Autodesk Inventor part; units mm, degrees
ref_plane "YZ Plane" through (0, 0, 0) normal (1, 0, 0) x (0, 1, 0)
ref_plane "XZ Plane" through (0, 0, 0) normal (0, 1, 0) x (-1, 0, 0)
ref_plane "XY Plane" through (0, 0, 0) normal (0, 0, 1) x (1, 0, 0)
sketch "Sketch1" plane through (0, 0, 0) normal (0, 1, 0) x (-1, 0, 0)
  line L0 (-29, 41.5) -> (29, 41.5)
  line L1 (29, 41.5) -> (29, -41.5)
  line L2 (29, -41.5) -> (-29, -41.5)
  line L3 (-29, -41.5) -> (-29, 41.5)
  line L4 (-29, 41.5) -> (29, -41.5) construction
  line L5 (29, 41.5) -> (-29, -41.5) construction
  point P0 (0, 0)
  dimension "d0" = 83
  dimension "d1" = 58
extrude "Extrusion1" add sketch "Sketch1" along normal blind 1.5
sketch "Sketch2" plane through (0, 1.5, 0) normal (0, 1, 0) x (1, 0, 0)
  line L0 (-29, 41.5) -> (-29, -41.5)
  point P0 (0, 0)
  point P1 (-24.75, 5.75)
  point P2 (-24.75, -4.25)
  point P3 (-29, 0)
  dimension "d11" = 10
  dimension "d12" = 4.25
  dimension "d13" = 4.25
  dimension "d14" = 5.75
hole "Hole1" at (-24.75, 1.5, -5.75) at (-24.75, 1.5, 4.25) direction (0, -1, 0) diameter 2 end through all
properties part number "pcb" material "PBT Plastic"
Read the model definition and answer for the solid it produces. Units are mm, in the model's axes. Coordinates: 2 decimals unless noted, no trailing zeros. Write each loop counter-clockwise with the first axis right and the second up, starting at its lowest first coordinate (ties: lowest second). Pieces come first, ordered by that corner, then holes. Notation, with made-up numbers: (-22.75, 23.25) - (12.25, 23.25) arc R27 ccw to (12.25, 58.25) - close; hole circle Ø4 at (35.5, 43.25). An arc over 180 degrees is marked (long way). Answer as a JSON object with one key per item and string values. Group by question number.
1. Consider L1, parallel to Z at x = -24.75, y = 0.65; L2, parallel to X at y = 0.7, z = 4.25. Determine where each line is inside the solid, lowest interval first. Write a range as [from, to].
2. The mould has two halves that part along Z. Classify faces 1 (the cylindrical face through (-23.774, 0.74, 4.033)), 2 (the cylindrical face through (-23.774, 0.74, -5.967)), 3 (the flat face through (0, 1.5, 1)): +Z half, -Z half, draft (parallel to the pull), parting line (faces both ways), or undercut.
3. A cutting plane is placed at A-A (z = -5.75). Determine the outline of the cut face in (x, y).
4. A cutting plane is placed at B-B (x = -24.75). Determine the outline of the cut face in (y, z).
Worked out:
{
 "1": {"L1": "z = [-41.5, -6.75], [-4.75, 3.25], [5.25, 41.5]", "L2": "x = [-29, -25.75], [-23.75, 29]"},
 "2": {"face 1": "undercut", "face 2": "undercut", "face 3": "draft"},
 "3": {"outline": "(-29, 0) - (-25.75, 0) - (-25.75, 1.5) - (-29, 1.5) - close; (-23.75, 0) - (29, 0) - (29, 1.5) - (-23.75, 1.5) - close"},
 "4": {"outline": "(0, -41.5) - (1.5, -41.5) - (1.5, -6.75) - (0, -6.75) - close; (0, -4.75) - (1.5, -4.75) - (1.5, 3.25) - (0, 3.25) - close; (0, 5.25) - (1.5, 5.25) - (1.5, 41.5) - (0, 41.5) - close"}
}
